Model file for the job. Use its own axes, mm. A direction names the side the tool comes from. Coordinates: 2 decimals unless noted, no trailing zeros. Order: outer loops, then holes, each group sorted by start corner. A loop starts at its lowest first (then second) coordinate and runs counter-clockwise, first axis right, second up.
from build123d import *

# Parameters (mm, degrees)
F0_W     = 31.75
F0_H     = 31.75
F1_DEPTH = 762
F2_R     = 3.175
F3_T     = -3.048
F4_R     = 4.5
F5_DEPTH = 15.875


with BuildPart() as f1:
    # F0 (on Top) → F1 (new body)
    with BuildSketch(Plane.XY):
        Rectangle(F0_W, F0_H)
    extrude(amount=-F1_DEPTH)

    # F2
    f2_edges = [f1.edges().sort_by_distance(p)[0] for p in [
        (-15.875, 15.875, -381),
        (-15.875, -15.875, -381),
        (15.875, 15.875, -381),
        (15.875, -15.875, -381),
    ]]
    fillet(f2_edges, radius=F2_R)

    # F3
    f3_openings = [f1.faces().sort_by_distance(p)[0] for p in [
        (0, 0, 0),
        (0, 0, -762),
    ]]
    offset(amount=F3_T, openings=f3_openings)

    # F4 (on Front) → F5 (cut, through all)
    with BuildSketch(Plane.XZ):
        with Locations((0, -38.1)):
            Circle(F4_R)
        with Locations((0, -635)):
            Circle(F4_R)
    extrude(amount=F5_DEPTH, mode=Mode.SUBTRACT)


solid = f1.part
Q1. Mould opens along Y. For faces 3 (the face through (0, -15.875, -376)), 4 (the face through (-15.875, 0, -376)), 5 (the face through (0, 12.827, -376)) say: pulls with the +Y half, pulls with the -Y half, needs draft (parallel to the pull), parting line crosses it, or undercut.
Established:
face 3: pulls with the -Y half
face 4: needs draft
face 5: undercut
Q2. Drop a flat-ended pin along its axis: P1, Ø4, axis at x = -6, y = 12, coming from the +Z side. Give the stop position or say it passes through.
Established:
P1: stops at z = 0
Q3. Cut at B-B, the plane z = -484. List the corners of the cut face in (x, y) (3 decimals), plus the area to 3 significant figures.
Established:
outline: (-15.875, -12.7) arc R3.175 ccw to (-12.7, -15.875) - (12.7, -15.875) arc R3.175 ccw to (15.875, -12.7) - (15.875, 12.7) arc R3.175 ccw to (12.7, 15.875) - (-12.7, 15.875) arc R3.175 ccw to (-15.875, 12.7) - close; hole (-12.827, -12.7) arc R0.127 ccw to (-12.7, -12.827) - (12.7, -12.827) arc R0.127 ccw to (12.827, -12.7) - (12.827, 12.7) arc R0.127 ccw to (12.7, 12.827) - (-12.7, 12.827) arc R0.127 ccw to (-12.827, 12.7) - close
area: 341 mm2
Q4. Which spindle directions (+Z, -Z, +X, -X, +Y, -Y) get a long thin tool onto all of the face, cutting with end or side? Do faces 1 (the face through (0, 15.875, -376)), 2 (the face through (-12.827, 0, -376)). Say none if no direction does.
Established:
face 1: +Z, -Z, +X, -X, +Y
face 2: +Z, -Z
Q5. Cut at A-A, the plane y = 1. List the corners of the cut face in (x, z) (3 decimals), plus the area to 3 significant figures.
Established:
outline: (-15.875, -762) - (-12.827, -762) - (-12.827, 0) - (-15.875, 0) - close; (12.827, -762) - (15.875, -762) - (15.875, 0) - (12.827, 0) - close
area: 4,650 mm2
Q6. Probe line 1 (Z direction, x = 0, y = -13); line 2 (X direction, y = -6, z = -594.5) (3 decimals). List the from-to ranges inside material, lowest first.
Established:
line 1: z = -762 to -639.5, -630.5 to -42.6, -33.6 to 0
line 2: x = -15.875 to -12.827, 12.827 to 15.875
